from build123d import *

# Parameters (mm, degrees)
BASE_EXTRUDE_DEPTH   = 15
SLOT_CUT_DEPTH       = 66.76473219
SKETCH3_R            = 5
GUIDE_HOLE_DEPTH     = 77.811457479
LPATTERN1_COUNT      = 3
LPATTERN1_PITCH      = 10
LPATTERN1_COUNT_DIR2 = 2
LPATTERN1_PITCH_DIR2 = 12
FILLET1_R            = 1


with BuildPart() as part:
    # Sketch1 → Base Extrude (new, symmetric)
    with BuildSketch(Plane.XY):
        Polygon((-50, 0), (50, 0), (50, 10), (19.558809371, 10), (5, 50), (-5, 50), (-19.558809371, 10), (-50, 10), align=None)
    extrude(amount=BASE_EXTRUDE_DEPTH, both=True)

    # Sketch2 → Slot Cut (cut, through all)
    with BuildSketch(Plane(origin=(0, 10, 0), x_dir=(1, 0, 0), z_dir=(0, 1, 0))):
        with BuildLine():
            Line((26, -5), (26, 5))
            ThreePointArc((26, 5), (30, 9), (34, 5))
            Line((34, 5), (34, -5))
            ThreePointArc((34, -5), (30, -9), (26, -5))
        make_face()
    slot_cut = extrude(amount=-SLOT_CUT_DEPTH, mode=Mode.SUBTRACT)

    # Mirror1: Slot Cut across plane
    add(slot_cut.mirror(Plane(origin=(0, 0, 0), x_dir=(0, 0, 1), z_dir=(1, 0, 0))), mode=Mode.SUBTRACT)

    # Sketch3 → Guide hole (cut, through all)
    with BuildSketch(Plane.XY.offset(15)):
        with Locations((0, 29)):
            Circle(SKETCH3_R)
    extrude(amount=-GUIDE_HOLE_DEPTH, mode=Mode.SUBTRACT)

    # Sketch10 → M3x0.5 Tapped Hole3 (revolve, cut)
    with BuildSketch(Plane(origin=(13.216501869, 27.425346647, 10), x_dir=(-0.3420201433256727, 0.939692620785907, 0), z_dir=(0, 0, 1))):
        Polygon((0, 0), (0, 8.251075774), (1.25, 7.5), (1.25, 0), align=None)
    m3x0_5_tapped_hole3 = revolve(axis=Axis((19.183550011, 29.597174557, 10), (-0.9396926207859069, -0.34202014332567277, 0)), mode=Mode.SUBTRACT)

    # LPattern1: M3x0.5 Tapped Hole3 3 × 2
    with Locations(*[Vector(0, 0, -1) * (i * LPATTERN1_PITCH) + Vector(0.34202014332567293, -0.9396926207859069, 0) * (j * LPATTERN1_PITCH_DIR2) for i in range(LPATTERN1_COUNT) for j in range(LPATTERN1_COUNT_DIR2) if (i, j) != (0, 0)]):
        add(m3x0_5_tapped_hole3, mode=Mode.SUBTRACT)

    # Fillet1
    fillet1_edges = [part.edges().sort_by_distance(p)[0] for p in [
        (-50, 10, 0),
        (-19.558809371, 10, 0),
        (19.558809371, 10, 0),
        (50, 10, 0),
    ]]
    fillet(fillet1_edges, radius=FILLET1_R)


solid = part.part
Source: CAD feature listing. Evaluate the final solid. Frame: model axes, mm. A direction names the side the tool comes from. Give positions to 0.01 mm unless a question says otherwise; leave off trailing zeros. Write each loop counter-clockwise with the first axis right and the second up, starting at its lowest first coordinate (ties: lowest second). Pieces come first, ordered by that corner, then holes. Notation, with made-up numbers: (-26, 47) -> (-16, 47) arc R26 ccw to (-16, 71) -> close; hole circle Ø5 at (32, 1). An arc over 180 degrees is marked (long way). Return JSON: item names as keys, results as strings. Group by question number.
1. Section D-D, the plane x = -32. Output: boundary loops of the cut face in (y, z).
2. Section A-A, the plane z = -3.5. Output: boundary loops of the cut face in (x, y), then the cut area to 3 significant figures.
3. Material intervals for line 1 (Y direction, x = 0, z = 6.25); line 2 (X direction, y = 31.5, z = -6); line 3 (Y direction, x = 36, z = 0), sorted ascending. Write a range as from..to.
4. Mould query, pull axis Z, two halves, no side actions, for faces 1 (the face through (-1, 14, -15)), 2 (the face through (12.26, 30.05, 0.21)), 3 (the face through (26, 5, 0)). Classes: +Z half, -Z half, draft (parallel to the pull), parting line (faces both ways), or undercut.
5. Section B-B, the plane x = 30. Output: boundary loops of the cut face in (y, z), then the cut area to 3 significant figures.
6. Access query for faces 4 (the face through (-50, 5, 0)), 5 (the face through (30, 5, 9)), 6 (the face through (5.517, 24.836, 0.083)), 7 (the face through (-34.4, 10, 0.2)). Directions: +Z, -Z, +X, -X, +Y, -Y. A direction counts if a zero-diameter tool reaches every point of the face in a straight line with its end or side. Return the directions, or none.
7. Section C-C, the plane y = 6. Output: boundary loops of the cut face in (x, z).
8. Pin query (flat end, axial travel): pin 1 Ø6 at (y, z) = (41, 2.5) entering from -X; pin 2 Ø8 at (x, y) = (18, 29.5) entering from +Z; pin 3 Ø2 at (x, z) = (-25.5, 10.5) entering from +Y; pin 4 Ø1.5 at (y, z) = (22, -0.5) entering from +X. Return the tip coordinate at first contact, or that it passes through.
Determined:
{
 "1": {"outline": "(0, -15) -> (10, -15) -> (10, -8.46) -> (0, -8.46) -> close; (0, 8.46) -> (10, 8.46) -> (10, 15) -> (0, 15) -> close"},
 "2": {"outline": "(-50, 0) -> (-34, 0) -> (-34, 10) -> (-49, 10) arc R1 ccw to (-50, 9) -> close; (-26, 0) -> (26, 0) -> (26, 10) -> (20.26, 10) arc R1 cw to (19.32, 10.66) -> (5, 50) -> (-5, 50) -> (-19.32, 10.66) arc R1 cw to (-20.26, 10) -> (-26, 10) -> close; (34, 0) -> (50, 0) -> (50, 9) arc R1 ccw to (49, 10) -> (34, 10) -> close; hole circle Ø10 at (0, 29)", "area": "1,740 mm2"},
 "3": {"line 1": "y = 0..24, 34..50", "line 2": "x = -11.73..-4.33, 4.33..11.73", "line 3": "y = 0..10"},
 "4": {"face 1": "-Z half", "face 2": "draft", "face 3": "undercut"},
 "5": {"outline": "(0, -15) -> (10, -15) -> (10, -9) -> (0, -9) -> close; (0, 9) -> (10, 9) -> (10, 15) -> (0, 15) -> close", "area": "120 mm2"},
 "6": {"face 4": "+Z, -Z, -X, +Y, -Y", "face 5": "+Y, -Y", "face 6": "none", "face 7": "+Z, -Z, -X, +Y"},
 "7": {"outline": "(-50, -15) -> (50, -15) -> (50, 15) -> (-50, 15) -> close; hole (-34, -5) arc R4 ccw to (-26, -5) -> (-26, 5) arc R4 ccw to (-34, 5) -> close; hole (26, -5) arc R4 ccw to (34, -5) -> (34, 5) arc R4 ccw to (26, 5) -> close"},
 "8": {"pin 1": "stops at x = -9.37", "pin 2": "passes through", "pin 3": "stops at y = 10", "pin 4": "stops at x = 15.46"}
}
